Check sheet for the modelled part. Datum: model origin and axes. Units: mm. A direction names the side the tool comes from. Coordinates: 2 decimals unless noted, no trailing zeros. Loops run counter-clockwise (first coordinate to the right, second up) from the corner with the lowest first, then second, coordinate; pieces in that order, holes last. Notation, with made-up numbers: M 76,55 L 132,55 A19 ccw 132,69 Z; hole C 38,-3.75 d9. An arc over 180 degrees is marked long. Return JSON: item names as keys, results as strings.
from build123d import *

# Parameters (mm, degrees)
F2_R          = 3
F3_DEPTH      = 6.001
F3_DEPTH_BACK = 6.001
F4_SIZE       = 0.5


with BuildPart() as f1:
    # F0 (on Front) → F1 (revolve)
    with BuildSketch(Plane.XZ):
        Polygon((0, 3.5), (0, 0), (72, 0), (72, 1), (60, 1), (60, 2), (52, 2), (52, 3.5), (42, 3.5), (42, 6), (10, 6), (10, 3.5), align=None)
    revolve(axis=Axis((37.3597331345, 0, 0), (1, 0, 0)))

    # F2 (on Top) → F3 (cut, two sides)
    with BuildSketch(Plane.XY) as f3_sk:
        with Locations((26, 0)):
            Circle(F2_R)
    extrude(amount=-F3_DEPTH, mode=Mode.SUBTRACT)
    extrude(f3_sk.sketch, amount=F3_DEPTH_BACK, mode=Mode.SUBTRACT)

    # F4
    f4_edges = [f1.edges().sort_by_distance(p)[0] for p in [
        (52, 0, -3.5),
        (0, 0, -3.5),
        (10, 0, -6),
        (42, 0, -6),
    ]]
    chamfer(f4_edges, length=F4_SIZE)


solid = f1.part
1) Go/stop test with flat-tipped pins: pin 1 Ø6 at (x, y) = (10.5, 0.5) entering from -Z; pin 2 Ø1.5 at (x, z) = (46.5, 4.5) entering from -Y; pin 3 Ø6 at (x, z) = (57.5, -4.5) entering from -Y; pin 4 Ø2 at (x, z) = (50.5, -2) entering from -Y. Record where each tip stops, or that it passes through.
Answers:
{"pin 1": "z = -6", "pin 2": "through", "pin 3": "y = -1.32", "pin 4": "y = -3.35"}
2) Section check B-B on x = 26. Record the cut outline in (y, z), then the cut area to 3 significant figures.
Answers:
{"outline": "M -3,-5.2 L -3,5.2 A6 ccw Z; M 3,-5.2 A6 ccw 3,5.2 Z", "area": "44.2 mm²"}
3) Set-up check for faces 1 (the face through (10, 0, 4)), 2 (the face through (72, 0, 0)), 3 (the face through (56, 2, 0)): record each of +Z, -Z, +X, -X, +Y, -Y from which the full face is reachable in a straight line by a thin tool's end or side.
Answers:
{"face 1": "-X", "face 2": "+Z, -Z, +X, +Y, -Y", "face 3": "+X"}
4) Section check C-C on x = 66. Record the cut outline in (y, z).
Answers:
{"outline": "C 0,0 d2"}
5) Scan lines: line 1 along X through (y, z) = (0, -3.75); line 2 along Y through (x, z) = (26, -3.25); line 3 along Y through (x, z) = (26, -4). Record each from-to range of solid material in increasing order. Write a range as [from, to].
Answers:
{"line 1": "[10, 23], [29, 42]", "line 2": "[-5.04, -3], [3, 5.04]", "line 3": "[-4.47, -3], [3, 4.47]"}
6) Section check D-D on x = 8. Record the cut outline in (y, z).
Answers:
{"outline": "C 0,0 d7"}
